Here's the drawing with two shaded views (mm, measured from the low corner). I have some questions. Round coordinates to 2 decimals unless told otherwise and drop trailing zeros. Loops run counter-clockwise (first coordinate to the right, second up) from the corner with the lowest first, then second, coordinate; pieces in that order, holes last. Notation, with made-up numbers: M 84,53.25 L 96,53.25 A27 cw 96,85.25 Z; hole C 78,-27 d5. An arc over 180 degrees is marked long. Answer as a JSON object with one key per item and string values.
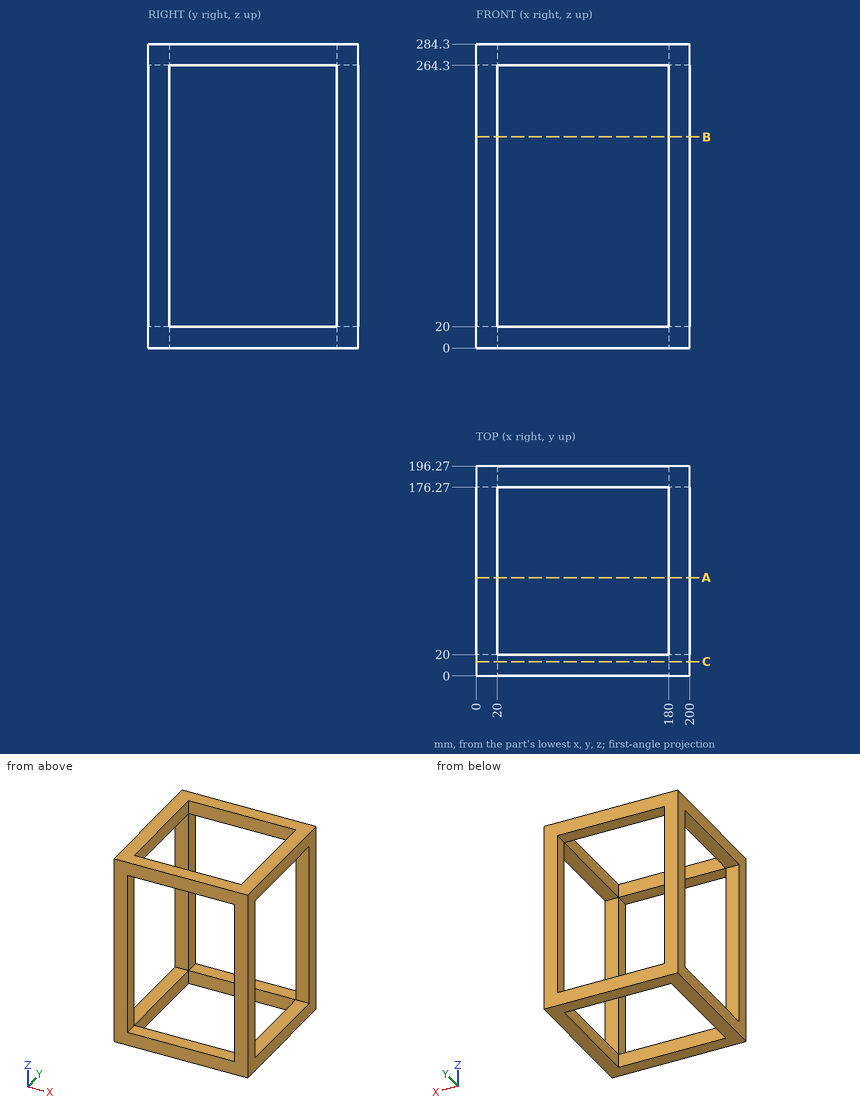
Item 1: If I drill on L1, parallel to Z at x = 191.5, y = 23; L2, parallel to Y at x = 35, z = 264.5; L3, parallel to X at y = 16, z = 41, over which ranges is the centre line in solid material (lowest first)? Write a range as from..to.
Solution:
{"L1": "z = 0..20, 264.3..284.3", "L2": "y = 0..20, 176.27..196.27", "L3": "x = 0..20, 180..200"}
Item 2: I want a section at C-C on y = 13.5. List the corners of the cut face in (x, z) for me, plus the area to 3 significant figures.
Solution:
{"outline": "M 0,0 L 200,0 L 200,284.3 L 0,284.3 Z; hole M 20,20 L 180,20 L 180,264.3 L 20,264.3 Z", "area": "17,800 mm2"}
Item 3: I want a section at A-A on y = 92. List the corners of the cut face in (x, z) for me.
Solution:
{"outline": "M 0,0 L 20,0 L 20,20 L 0,20 Z; M 0,264.3 L 20,264.3 L 20,284.3 L 0,284.3 Z; M 180,0 L 200,0 L 200,20 L 180,20 Z; M 180,264.3 L 200,264.3 L 200,284.3 L 180,284.3 Z"}
Item 4: For P1, Ø22, axis at x = 135, y = 10, coming from the -Z side, with a flat end and sliding along its axis, tell me the tip position at first contact or that it passes through.
Solution:
{"P1": "stops at z = 0"}
Item 5: I want a section at B-B on z = 197.5. List the corners of the cut face in (x, y) for me.
Solution:
{"outline": "M 0,0 L 20,0 L 20,20 L 0,20 Z; M 0,176.27 L 20,176.27 L 20,196.27 L 0,196.27 Z; M 180,0 L 200,0 L 200,20 L 180,20 Z; M 180,176.27 L 200,176.27 L 200,196.27 L 180,196.27 Z"}
